The figure shows three views and two pictorial views of one solid part (mm, origin at its lowest corner). Answer the questions. A direction names the side the tool comes from. Coordinates: 2 decimals unless noted, no trailing zeros. Loops run counter-clockwise (first coordinate to the right, second up) from the corner with the lowest first, then second, coordinate; pieces in that order, holes last.
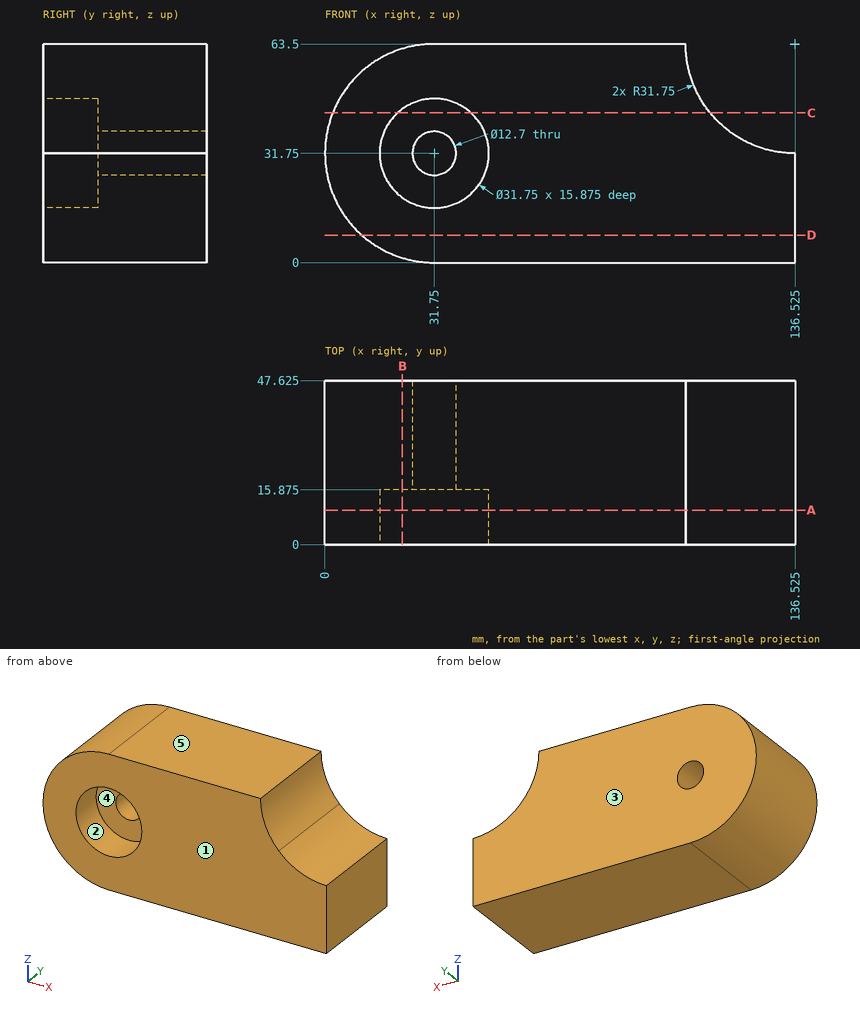
Q1. A cutting plane is placed at D-D (z = 8). Give the vertices of the cut face in (x, y) (3 decimals).
Findings below:
outline: (10.679, 0) - (136.525, 0) - (136.525, 47.625) - (10.679, 47.625) - close
Q2. Determine the mould class of the marked faces 3, 4 and 5 for opening direction Z: +Z half, -Z half, draft (parallel to the pull), parting line (faces both ways), or undercut.
Findings below:
face 3: draft
face 4: undercut
face 5: +Z half
Q3. Which of the six approach directions +Z, -Z, +X, -X, +Y, -Y give full straight-line access (tool end or side, diameter ignored) to the marked faces 1 and 2?
Findings below:
face 1: +Z, -Z, +X, -X, -Y
face 2: -Y
Q4. Flat-ended cylindrical pins translate along their axes: pin 1 Ø5 at (x, y) = (79.5, 39) entering from -Z; pin 2 Ø10 at (x, z) = (113.5, 56.5) entering from +Y; pin 3 Ø1.5 at (x, z) = (18.5, 34) entering from -Y (3 decimals). Find the tip coordinate at first contact, or state that the pin passes through.
Findings below:
pin 1: stops at z = 0
pin 2: passes through
pin 3: stops at y = 15.875
Q5. A cutting plane is placed at A-A (y = 10). Give the vertices of the cut face in (x, z) (3 decimals).
Findings below:
outline: (31.75, 0) - (136.525, 0) - (136.525, 31.75) arc R31.75 cw to (113.608, 41.525) arc R31.75 cw to (104.775, 63.5) - (31.75, 63.5) arc R31.75 ccw to start; hole circle Ø31.75 at (31.75, 31.75)
Q6. Straight lines are drawn through the part: probe 1 along Z at (x, y) = (31.75, 37); probe 2 along X at (y, z) = (33.5, 31.5) (3 decimals); probe 3 along Z at (x, y) = (31.75, 9) (3 decimals). For each, find the intervals that lie inside material, in ascending order.
Findings below:
probe 1: z = 0 to 25.4, 38.1 to 63.5
probe 2: x = 0.001 to 25.405, 38.095 to 136.525
probe 3: z = 0 to 15.875, 47.625 to 63.5
Q7. A cutting plane is placed at C-C (z = 43.5). Give the vertices of the cut face in (x, y) (3 decimals).
Findings below:
outline: (2.254, 0) - (21.075, 0) - (21.075, 15.875) - (42.425, 15.875) - (42.425, 0) - (111.866, 0) - (111.866, 47.625) - (2.254, 47.625) - close
Q8. A cutting plane is placed at B-B (x = 22.5). Give the vertices of the cut face in (y, z) (3 decimals), then the cut area to 3 significant figures.
Findings below:
outline: (0, 1.377) - (47.625, 1.377) - (47.625, 62.123) - (0, 62.123) - (0, 44.652) - (15.875, 44.652) - (15.875, 18.848) - (0, 18.848) - close
area: 2,480 mm2
